Autodesk Fusion 360 part; units mm, degrees
sketch "Sketch1" plane through (0, 0, 0) normal (0, 1, 0) x (1, 0, 0)
  line L0 (30, 12.5) -> (-30, 12.5)
  line L1 (-30, 12.5) -> (-30, -12.5)
  line L2 (-30, -12.5) -> (30, -12.5)
  line L3 (30, -12.5) -> (30, 12.5)
  line L4 (30, 12.5) -> (-30, -12.5) construction
  line L5 (-30, 12.5) -> (30, -12.5) construction
  line L6 (-30, -12.5) -> (-50, -12.5)
  line L7 (-50, -12.5) -> (-50, -10.5)
  line L8 (-50, -10.5) -> (-32, -10.5)
  line L9 (-32, -10.5) -> (-32, 14.5)
  line L10 (-32, 14.5) -> (32, 14.5)
  line L11 (32, 14.5) -> (32, -10.5)
  line L12 (32, -10.5) -> (50, -10.5)
  line L13 (50, -10.5) -> (50, -12.5)
  line L14 (50, -12.5) -> (30, -12.5)
  dimension "d1" = 60
  dimension "d2" = 25
  dimension "d3" = 20
  dimension "d4" = 2
  dimension "d6" = 18
  dimension "d7" = 25
  dimension "d8" = 64
  dimension "d9" = 25
  dimension "d10" = 2
extrude "Extrude1" add sketch "Sketch1" along normal blind 70 contours L0 L1 L3 L6 L7 L8 L9 L10 L11 L12 L13 L14
sketch "Sketch2" plane through (0, 0, -14.5) normal (0, 0, -1) x (-1, 0, 0)
  line L0 (-32, 0) -> (32, 0)
  line L1 (32, 0) -> (32, 70)
  line L2 (32, 70) -> (-32, 70)
  line L3 (-32, 70) -> (-32, 0)
  line L4 (0, 70) -> (0, 0) construction
  line L5 (0, 70) -> (0, 54.76) construction
  line L6 (0, 54.76) -> (0, 56.03)
  line L7 (0, 56.03) -> (24.257, 56.03) construction
  line L8 (0, 54.76) -> (-24.13, 54.76) construction
  circle A0 centre (-24.13, 54.76) radius 1.6
  circle A1 centre (24.257, 56.03) radius 1.6
  line L9 (-24.13, 54.76) -> (-24.13, 3.96) construction
  line L10 (-24.13, 3.96) -> (-8.89, 3.96) construction
  circle A2 centre (-8.89, 3.96) radius 1.6
  line L11 (-8.89, 3.96) -> (19.05, 3.96) construction
  circle A3 centre (19.05, 3.96) radius 1.6
  circle A4 centre (-24.13, 54.76) radius 3.2
  circle A5 centre (24.257, 56.03) radius 3.2
  line L12 (-14, 10) -> (14, 10)
  line L13 (22, 18) -> (22, 52)
  line L14 (14, 60) -> (-14, 60)
  line L15 (-22, 52) -> (-22, 18)
  arc A6 (-14, 60) -> (-22, 52) centre (-14, 52) ccw
  arc A7 (22, 52) -> (14, 60) centre (14, 52) ccw
  arc A8 (14, 10) -> (22, 18) centre (14, 18) ccw
  arc A9 (-22, 18) -> (-14, 10) centre (-14, 18) ccw
  dimension "d13" = 15.24
  dimension "d16" = 1.27
  dimension "d19" = 24.257
  dimension "d20" = 24.13
  dimension "d21" = 3.2
  dimension "d22" = 3.2
  dimension "d23" = 50.8
  dimension "d24" = 15.24
  dimension "d25" = 3.2
  dimension "d26" = 27.94
  dimension "d27" = 3.2
  dimension "d41" = 6.4
  dimension "d42" = 6.4
  dimension "d44" = 8
  dimension "d45" = 8
  dimension "d46" = 8
  dimension "d47" = 8
extrude "Extrude4" cut sketch "Sketch2" against normal blind 2 contours A4 A5 L12 L13 L14 L15 A6 A7 A8 A9
extrude "Extrude2" cut sketch "Sketch2" against normal blind 2 contours A0 | A1 | A2 | A3
fillet "Fillet1" radius 10 4 edges at (-50, 70, 11.5) (50, 70, 11.5) (50, 0, 11.5) (-50, 0, 11.5)
fillet "Fillet2" radius 2 8 edges at (-30, 35, 12.5) (-30, 35, -12.5) (30, 35, -12.5) (30, 35, 12.5) (32, 35, 10.5) (32, 35, -14.5) (-32, 35, -14.5) (-32, 35, 10.5)
sketch "Sketch3" plane through (0, 0, 12.5) normal (0, 0, 1) x (1, 0, 0)
  line L0 (32, 70) -> (32, 0)
  line L1 (32, 0) -> (40, 0)
  arc A0 (40, 0) -> (50, 10) centre (40, 10) ccw
  line L2 (50, 10) -> (50, 60)
  arc A1 (50, 60) -> (40, 70) centre (40, 60) ccw
  line L3 (40, 70) -> (32, 70)
  circle A2 centre (40, 60) radius 2
  circle A3 centre (40, 10) radius 2
  line L4 (0, 0) -> (0, 70) construction
  line L5 (40, 60) -> (-40, 60) construction
  line L6 (40, 10) -> (-40, 10) construction
  circle A4 centre (-40, 60) radius 2
  circle A5 centre (-40, 10) radius 2
  dimension "d32" = 4
  dimension "d33" = 4
  dimension "d34" = 80
  dimension "d35" = 80
  dimension "d36" = 4
  dimension "d37" = 4
extrude "Extrude3" cut sketch "Sketch3" against normal blind 2 contours A2 | A3 | A4 | A5
equation "d4 = width"
equation "width = 2 mm"
equation "d6 = 20 mm - width"
equation "d8 = 60 mm + 2 * width"
equation "d10 = width"
The listing builds one solid part. Answer for the finished solid, in the listing's coordinates (mm). A direction names the side the tool comes from. Round coordinates to 2 decimals unless told otherwise and drop trailing zeros. Loops run counter-clockwise (first coordinate to the right, second up) from the corner with the lowest first, then second, coordinate; pieces in that order, holes last. Notation, with made-up numbers: (37, 64) -> (81, 64) arc R16 ccw to (81, 78) -> close; hole circle Ø5 at (6, -15.5). An arc over 180 degrees is marked (long way). Use one line per item in the form item = value.
1. A tool of negligible diameter and unlimited length cuts with its end or side. For faces 5 (the flat face through (-42, 35, 10.5)), 6 (the cylindrical face through (46.99, 2.85, 11.51)), 7 (the flat face through (-30, 35, 0)), 8 (the flat face through (41, 35, 12.5)), 9 (the cylindrical face through (-19.594, 12.281, -13.514)), from which of +Z, -Z, +X, -X, +Y, -Y can it reach the whole face along a straight path? Write none if from no direction.
Answer key:
face_5 = -Z, -X, +Y, -Y
face_6 = +Z, -Z, +X, -Y
face_7 = +Z, +Y, -Y
face_8 = +Z, +X, -X, +Y, -Y
face_9 = +Z, -Z
2. The part is cut by section A-A on x = 1.5. Determine the outline of the cut face in (y, z), and give its area (3 significant figures).
Answer key:
outline = (0, -14.5) -> (10, -14.5) -> (10, -12.5) -> (0, -12.5) -> close; (60, -14.5) -> (70, -14.5) -> (70, -12.5) -> (60, -12.5) -> close
area = 40.0 mm²
3. The part is cut by section C-C on y = 21. Determine the outline of the cut face in (x, z), and give its area (3 significant figures).
Answer key:
outline = (-50, 10.5) -> (-34, 10.5) arc R2 cw to (-32, 8.5) -> (-32, -12.5) arc R2 ccw to (-30, -14.5) -> (-22, -14.5) -> (-22, -12.5) -> (-28, -12.5) arc R2 cw to (-30, -10.5) -> (-30, 10.5) arc R2 ccw to (-32, 12.5) -> (-50, 12.5) -> close; (22, -14.5) -> (30, -14.5) arc R2 ccw to (32, -12.5) -> (32, 8.5) arc R2 cw to (34, 10.5) -> (50, 10.5) -> (50, 12.5) -> (32, 12.5) arc R2 ccw to (30, 10.5) -> (30, -10.5) arc R2 cw to (28, -12.5) -> (22, -12.5) -> close
area = 212 mm²
4. The part is cut by section D-D on x = -19. Determine the outline of the cut face in (y, z) (3 decimals), and give its area (3 significant figures).
Answer key:
outline = (0, -14.5) -> (2.361, -14.5) -> (2.361, -12.5) -> (0, -12.5) -> close; (5.559, -14.5) -> (11.755, -14.5) -> (11.755, -12.5) -> (5.559, -12.5) -> close; (58.245, -14.5) -> (70, -14.5) -> (70, -12.5) -> (58.245, -12.5) -> close
area = 40.6 mm²
5. Find the intervals of material crossed by probe 1 along Y at (x, z) = (40, 11.8); probe 2 along X at (y, z) = (52, 8); probe 3 along Y at (x, z) = (-19.05, -14.1), in increasing order. Write a range as [from, to].
Answer key:
probe_1 = [0, 8], [12, 58], [62, 70]
probe_2 = [-32, -30], [30, 32]
probe_3 = [0, 2.36], [5.56, 11.8], [58.2, 70]
6. For a pull along Y with two mould halves and no side action, classify faces 1 (the flat face through (-22, 35, -14)), 2 (the flat face through (0, 70, -13)), 3 (the cylindrical face through (-41.474, 11.352, 11.514)), 4 (the cylindrical face through (-31.4, 35.49, -13.93)) as released by +Y, released by -Y, zero draft, split by the parting line, or undercut.
Answer key:
face_1 = undercut
face_2 = released by +Y
face_3 = undercut
face_4 = zero draft
7. Flat-ended cylindrical pins translate along their axes: pin 1 Ø5 at (x, y) = (-40, 10) entering from -Z; pin 2 Ø6.5 at (y, z) = (49, 2.5) entering from +X; pin 3 Ø0.6 at (y, z) = (31, -13.5) entering from +X; pin 4 Ø10 at (x, y) = (13, 31) entering from +Z. Find the tip coordinate at first contact, or state that the pin passes through.
Answer key:
pin_1 = 10.5
pin_2 = 32
pin_3 = 31.87
pin_4 = through
8. The part is cut by section B-B on z = -6. Determine the outline of the cut face in (x, y), and give its area (3 significant figures).
Answer key:
outline = (-32, 0) -> (-30, 0) -> (-30, 70) -> (-32, 70) -> close; (30, 0) -> (32, 0) -> (32, 70) -> (30, 70) -> close
area = 280 mm²
